Work out the finished part from the listing and answer in its coordinate system (mm). Coordinates: 2 decimals unless noted, no trailing zeros. Write each loop counter-clockwise with the first axis right and the second up, starting at its lowest first coordinate (ties: lowest second). Pieces come first, ordered by that corner, then holes. Notation, with made-up numbers: (40, 47) - (56, 47) arc R25 cw to (56, 70) - close; hole circle Ø11 at (12.5, 67). An arc over 180 degrees is marked (long way). Use one line per item in the form item = value. Start each with the question number.
Item 1: Given pin 1 (10 mm diameter, centred on y = 9, z = 17.5, fed in from -X); pin 2 (5 mm diameter, centred on y = -0.5, z = 10.5, fed in from +X); pin 3 (1.5 mm diameter, centred on y = 14, z = 14, fed in from -X), each flat-ended and moving along its own axis, determine where each tip first touches the part or whether it passes through.
Item 2: Consider probe 1 along Y at (x, z) = (0, 16.5); probe 2 along Y at (x, z) = (-4, 6); probe 3 along X at (y, z) = (12, 15.5). Determine where each line is inside the solid, lowest interval first.
Item 3: A cutting plane is placed at C-C (z = 5.25). Write down the section's boundary in (x, y).
Item 4: A cutting plane is placed at D-D (x = 19.5). Write down the section's boundary in (y, z), then the cut area to 3 significant figures.
Item 5: Determine the mould class of faces 1 (the flat face through (0, 21.218, 10)), 2 (the flat face through (18.46, 10.46, 10.16)), 3 (the cylindrical face through (12.83, 4.04, 10.44)) for opening direction X: released by +X, released by -X, zero draft, split by the parting line, or undercut.
Item 6: A cutting plane is placed at B-B (y = -6). Write down the section's boundary in (x, z), then the cut area to 3 significant figures.
Item 7: A cutting plane is placed at A-A (x = 0). Write down the section's boundary in (y, z), then the cut area to 3 significant figures.
from build123d import *

# Parameters (mm, degrees)
F1_DEPTH  = 20.6
F2_R      = 13.45
F3_DEPTH  = 25
F3_FACE_R = 13.45
F4_DEPTH  = 45.601


with BuildPart() as f1:
    # F0 (on Top) → F1 (new body)
    with BuildSketch(Plane.XY):
        Polygon((-12.25, -21.217622), (12.25, -21.217622), (24.5, 0), (12.25, 21.217622), (-12.25, 21.217622), (-24.5, 0), align=None)
    extrude(amount=F1_DEPTH)

    # F2 (on face) → F3 (join)
    with BuildSketch(Plane.XY.offset(20.6)):
        Circle(F2_R)
    extrude(amount=F3_DEPTH)

    # F3_face (on face) → F4 (cut, through all)
    with BuildSketch(Plane.XY.offset(45.6)):
        Circle(F3_FACE_R)
    extrude(amount=-F4_DEPTH, mode=Mode.SUBTRACT)


solid = f1.part
Answer:
q1.pin_1 = -22.19
q1.pin_2 = 24.5
q1.pin_3 = -16.85
q2.probe_1 = -21.22 to -13.45, 13.45 to 21.22
q2.probe_2 = -21.22 to -12.84, 12.84 to 21.22
q2.probe_3 = -17.57 to -6.07, 6.07 to 17.57
q3.outline = (-24.5, 0) - (-12.25, -21.22) - (12.25, -21.22) - (24.5, 0) - (12.25, 21.22) - (-12.25, 21.22) - close; hole circle Ø26.9 at (0, 0)
q4.outline = (-8.66, 0) - (8.66, 0) - (8.66, 20.6) - (-8.66, 20.6) - close
q4.area = 357 mm²
q5.face_1 = zero draft
q5.face_2 = released by +X
q5.face_3 = undercut
q6.outline = (-21.04, 0) - (-12.04, 0) - (-12.04, 20.6) - (-21.04, 20.6) - close; (12.04, 0) - (21.04, 0) - (21.04, 20.6) - (12.04, 20.6) - close
q6.area = 371 mm²
q7.outline = (-21.22, 0) - (-13.45, 0) - (-13.45, 20.6) - (-21.22, 20.6) - close; (13.45, 0) - (21.22, 0) - (21.22, 20.6) - (13.45, 20.6) - close
q7.area = 320 mm²
